Read the model definition and answer for the solid it produces. Units are mm, in the model's axes. A direction names the side the tool comes from. Coordinates: 2 decimals unless noted, no trailing zeros. Loops run counter-clockwise (first coordinate to the right, second up) from the corner with the lowest first, then second, coordinate; pieces in that order, holes last. Notation, with made-up numbers: M 60,51 L 64,51 A21 cw 64,89 Z; hole C 20,23 d7. An arc over 180 degrees is marked long. Put each result on its own line as item: value.
from build123d import *

# Parameters (mm, degrees)
F0_W     = 20
F0_H     = 9.45
F1_DEPTH = 10
F2_W     = 20
F2_H     = 3
F3_DEPTH = 3.3


with BuildPart() as f1:
    # F0 (on Front) → F1 (new body)
    with BuildSketch(Plane.XZ):
        with Locations((10, 4.725)):
            Rectangle(F0_W, F0_H)
    extrude(amount=F1_DEPTH)

    # F2 (on Top) → F3 (cut)
    with BuildSketch(Plane.XY):
        with Locations((10, -8.5)):
            Rectangle(F2_W, F2_H)
        with Locations((10, -1.5)):
            Rectangle(F2_W, F2_H)
    extrude(amount=F3_DEPTH, mode=Mode.SUBTRACT)


solid = f1.part
1) Find section C-C, the plane y = -2. Write down the section's boundary in (x, z).
Answer list:
outline: M 0,3.3 L 20,3.3 L 20,9.45 L 0,9.45 Z
2) Which of the six approach directions +Z, -Z, +X, -X, +Y, -Y give full straight-line access (tool end or side, diameter ignored) to faces 1 (the flat face through (10, -10, 6)), 2 (the flat face through (10, -3, 2)), 3 (the flat face through (10, -8, 3.3))?
Answer list:
face 1: +Z, -Z, +X, -X, -Y
face 2: -Z, +X, -X, +Y
face 3: -Z, +X, -X, -Y
3) Straight lines are drawn through the part: line 1 (Y direction, x = 10, z = 2.5); line 2 (Z direction, x = 12.5, y = -0.25). For each, find the intervals that lie inside material, in ascending order. Write a range as [from, to].
Answer list:
line 1: y = [-7, -3]
line 2: z = [3.3, 9.45]
4) Find section A-A, the plane x = 2.5. Write down the section's boundary in (y, z).
Answer list:
outline: M -10,3.3 L -7,3.3 L -7,0 L -3,0 L -3,3.3 L 0,3.3 L 0,9.45 L -10,9.45 Z
5) Find section B-B, the plane z = 3. Write down the section's boundary in (x, y).
Answer list:
outline: M 0,-7 L 20,-7 L 20,-3 L 0,-3 Z
6) Given pin 1 Ø2 at (x, z) = (5, 3) entering from -Y; pin 2 Ø2.5 at (x, y) = (15, -9) entering from -Z; pin 3 Ø1 at (x, z) = (15.5, 1.5) entering from -Y, each flat-ended and moving along its own axis, determine where each tip first touches the part or whether it passes through.
Answer list:
pin 1: stops at y = -10
pin 2: stops at z = 3.3
pin 3: stops at y = -7
